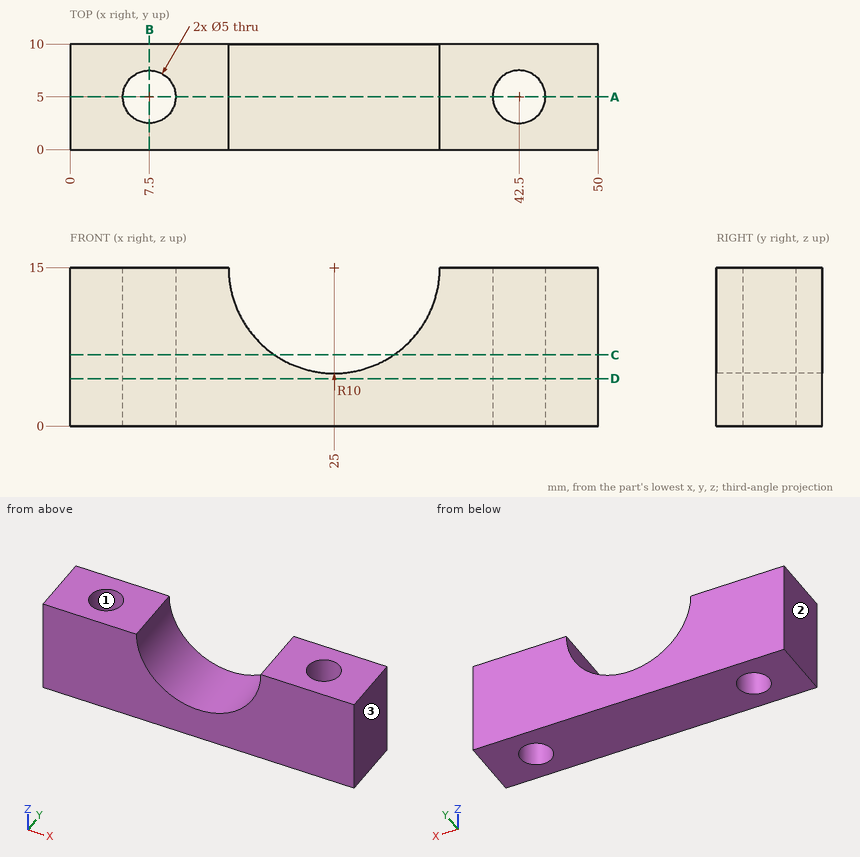
Could you check a few things on this drawing? It's one solid part, dimensions in mm from its lowest x, y, z. Coordinates: 2 decimals unless noted, no trailing zeros. Order: outer loops, then holes, each group sorted by start corner. A loop starts at its lowest first (then second) coordinate and runs counter-clockwise, first axis right, second up.
1. If we section it at D-D (z = 4.5): Please give me the cut outline in (x, y), then the cut area to 3 significant figures.
2. If we section it at C-C (z = 6.75): Please give me the cut outline in (x, y), then the cut area to 3 significant figures.
3. If we section it at B-B (x = 7.5): Please give me the cut outline in (y, z).
4. I need wall thicknesses on line 1 (X direction, y = 6.25, z = 7.5); line 2 (Y direction, x = 7.5, z = 10.75); line 3 (X direction, y = 2.25, z = 11.25). Which ranges of each line are inside material? Lowest first, please.
5. I'm going to push a flat-ended pin straight in: pin 1 (4 mm diameter, centred on x = 36.5, z = 9.5, fed in from -Y). Where does the tip first touch, or does it pass through?
6. If we section it at A-A (y = 5): Please give me the cut outline in (x, z).
7. Thinking about a two-plate mould opening in X: for the marked faces 1, 2 and 3, which applies, +X half, -X half, draft (parallel to the pull), parting line (faces both ways), or undercut?
Entries:
1. outline: (0, 0) - (50, 0) - (50, 10) - (0, 10) - close; hole circle Ø5 at (7.5, 5); hole circle Ø5 at (42.5, 5)
1. area: 461 mm2
2. outline: (0, 0) - (19.35, 0) - (19.35, 10) - (0, 10) - close; (30.65, 0) - (50, 0) - (50, 10) - (30.65, 10) - close; hole circle Ø5 at (7.5, 5); hole circle Ø5 at (42.5, 5)
2. area: 348 mm2
3. outline: (0, 0) - (2.5, 0) - (2.5, 15) - (0, 15) - close; (7.5, 0) - (10, 0) - (10, 15) - (7.5, 15) - close
4. line 1: x = 0 to 5.33, 9.67 to 18.39, 31.61 to 40.33, 44.67 to 50
4. line 2: y = 0 to 2.5, 7.5 to 10
4. line 3: x = 0 to 15.73, 34.27 to 50
5. pin 1: stops at y = 0
6. outline: (0, 0) - (5, 0) - (5, 15) - (0, 15) - close; (10, 0) - (40, 0) - (40, 15) - (35, 15) arc R10 cw to (15, 15) - (10, 15) - close; (45, 0) - (50, 0) - (50, 15) - (45, 15) - close
7. face 1: undercut
7. face 2: -X half
7. face 3: +X half
